Source: three-view drawing plus pictorial views. Frame: mm from the lowest corner of the part. A direction names the side the tool comes from. Round coordinates to 2 decimals unless told otherwise and drop trailing zeros. Loops run counter-clockwise (first coordinate to the right, second up) from the corner with the lowest first, then second, coordinate; pieces in that order, holes last. Notation, with made-up numbers: M 24.5,27 L 67.5,27 A13 ccw 67.5,32 Z; hole C 50.5,-6.75 d3. An arc over 180 degrees is marked long. Return JSON: item names as keys, results as strings. Group by question number.
1) Material intervals for line 1 (Y direction, x = 80, z = 330); line 2 (X direction, y = 30, z = 342); line 3 (X direction, y = 41, z = 251), sorted ascending. Write a range as from..to.
2) Contact query for flat-ended pins moving along their axis: P1, Ø6, axis at x = 73.5, z = 316, coming from the -Y side; P2, Ø12, axis at x = 66.5, y = 62, coming from the +Z side; P3, Ø10, axis at y = 16.5, z = 101, coming from the +X side. Output: stop coordinate, or through.
3) Section B-B (z = 225.5). Output: boundary loops of the cut face in (x, y), plus the area to 3 significant figures.
4) Section A-A (z = 35.5). Output: boundary loops of the cut face in (x, y), plus the area to 3 significant figures.
5) Access query for the marked faces 1 and 2. Directions: +Z, -Z, +X, -X, +Y, -Y. A direction counts if a zero-diameter tool reaches every point of the face in a straight line with its end or side. Return the directions, or none.
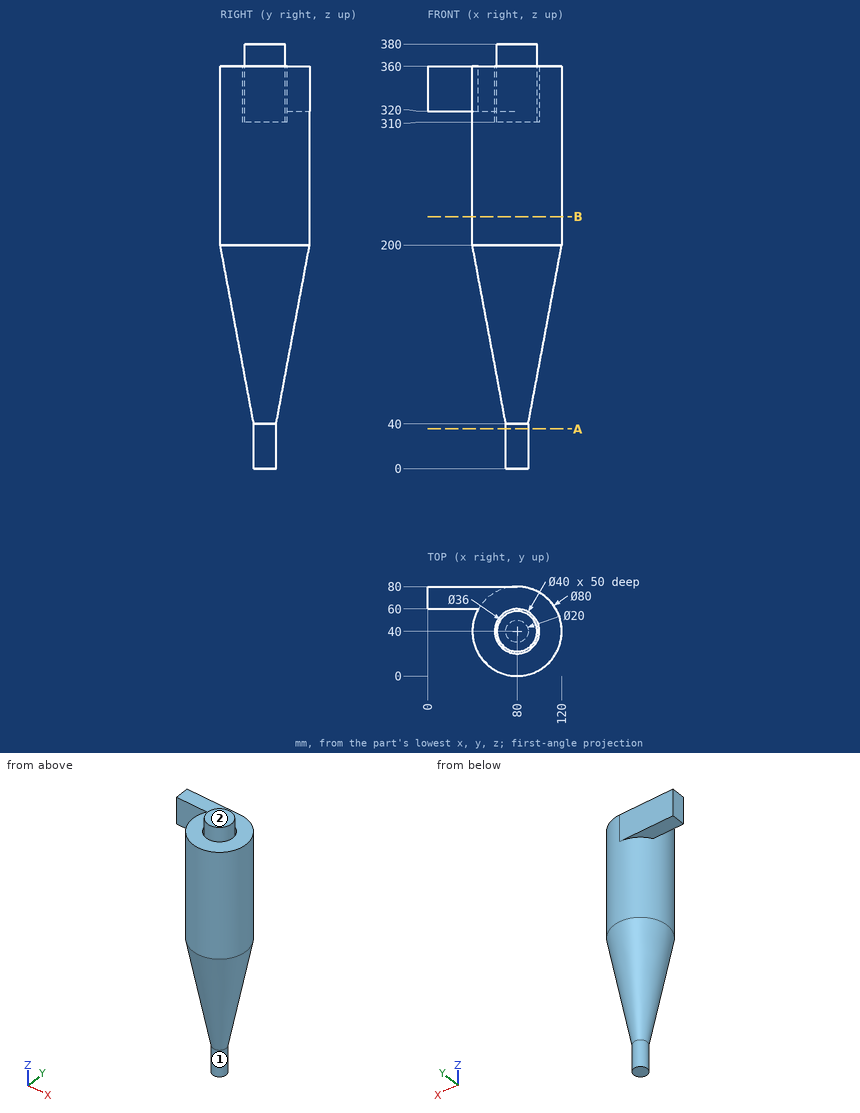
Returned:
{
 "1": {"line 1": "y = 0..20, 22..58, 60..80", "line 2": "x = 41.27..62.68, 65.03..94.97, 97.32..118.73", "line 3": "x = 40.01..119.99"},
 "2": {"P1": "stops at y = 0.15", "P2": "stops at z = 360", "P3": "stops at x = 91.03"},
 "3": {"outline": "C 80,40 d80", "area": "5,030 mm^2"},
 "4": {"outline": "C 80,40 d20", "area": "314 mm^2"},
 "5": {"face 1": "-Z", "face 2": "+Z, +X, -X, +Y, -Y"}
}
